Check sheet for the modelled part. Datum: model origin and axes. Units: mm. A direction names the side the tool comes from. Round coordinates to 2 decimals unless told otherwise and drop trailing zeros. Write each loop counter-clockwise with the first axis right and the second up, starting at its lowest first coordinate (ties: lowest second). Pieces come first, ordered by that corner, then holes.
Item 1: Release check for a two-part mould opening along X. For faces 1 (the cylindrical face through (-2.532, -59.947, 12.325)), 2 (the flat face through (0, 51.337, 12)), 3 (the flat face through (39, -13, 25)) record: pulls with the +X half, pulls with the -X half, needs draft (parallel to the pull), parting line crosses it, or undercut.
Item 2: Material ranges on line 1 along Y through (x, z) = (0, 10); line 2 along Y through (x, z) = (-31.5, 21.75); line 3 along X through (y, z) = (-3, 8), recorded low to high.
Item 3: Depth check by flat-ended pin: pin 1 (1.5 mm diameter, centred on y = 45.5, z = 22.5, fed in from -X); pin 2 (3 mm diameter, centred on x = 31, y = 26, fed in from -Z); pin 3 (1.5 mm diameter, centred on y = -29, z = 19.5, fed in from +X); pin 4 (10 mm diameter, centred on y = 35.5, z = 15, fed in from -X). Enter the tip coordinate at first touch or a pass-through.
Item 4: Section check B-B, the plane x = 0. Record the cut outline in (y, z).
Item 5: Section check D-D, the plane y = -49.5. Record the cut outline in (x, z), plus the area to 3 significant figures.
Item 6: Section check A-A, the plane y = 0. Record the cut outline in (x, z).
Item 7: Section check C-C, the plane z = 2. Record the cut outline in (x, y), plus the area to 3 significant figures.
Item 8: Set-up check for faces 4 (the cylindrical face through (-8.67, -39.05, 12.32)), 5 (the flat face through (-5.97, 56.05, 12.32)): record each of +Z, -Z, +X, -X, +Y, -Y from which the full face is reachable in a straight line by a thin tool's end or side.
from build123d import *

# Parameters (mm, degrees)
F0_R     = 60
F0_R_2   = 40
F1_DEPTH = 25
F4_DEPTH = 25.001


with BuildPart() as f1:
    # F0 (on Top) → F1 (new body)
    with BuildSketch(Plane.XY):
        Circle(F0_R)
        Circle(F0_R_2, mode=Mode.SUBTRACT)
    extrude(amount=F1_DEPTH)

    # F3 (on Top) + F2 (on face) → F4 (cut, through all)
    with BuildSketch(Plane.XY):
        with BuildLine():
            ThreePointArc((7.58927, 59.51809), (0, 60.215254), (-7.58927, 59.51809))
            Line((-7.58927, 59.51809), (-4.312616, 52.491282))
            ThreePointArc((-4.312616, 52.491282), (-3.574599, 51.649735), (-2.5, 51.336518))
            Line((-2.5, 51.336518), (2.5, 51.336518))
            ThreePointArc((2.5, 51.336518), (3.574599, 51.649735), (4.312616, 52.491282))
            Line((4.312616, 52.491282), (7.58927, 59.51809))
        make_face()
    with BuildSketch(Plane(origin=(0, 0, 0), x_dir=(1, 0, 0), z_dir=(0, 0, -1))):
        with BuildLine():
            Line((-3.065543, -69.518532), (0, -60))
            ThreePointArc((0, -60), (-11.359106, -58.914945), (-22.307369, -55.699024))
            Line((-22.307369, -55.699024), (-22.307369, -65.699024))
            ThreePointArc((-22.307369, -65.699024), (-14.254384, -75.507649), (-3.065543, -69.518532))
        make_face()
    extrude(amount=F4_DEPTH, mode=Mode.SUBTRACT)


solid = f1.part
Values found:
1. face 1: parting line crosses it
1. face 2: undercut
1. face 3: needs draft
2. line 1: y = -60 to -40, 40 to 51.34
2. line 2: y = -51.07 to -24.65, 24.65 to 51.07
2. line 3: x = -59.92 to -39.89, 39.89 to 59.92
3. pin 1: stops at x = -39.97
3. pin 2: stops at z = 0
3. pin 3: stops at x = 52.93
3. pin 4: stops at x = -51.67
4. outline: (-60, 0) - (-40, 0) - (-40, 25) - (-60, 25) - close; (40, 0) - (51.34, 0) - (51.34, 25) - (40, 25) - close
5. outline: (-33.91, 0) - (33.91, 0) - (33.91, 25) - (-33.91, 25) - close
5. area: 1,700 mm2
6. outline: (-60, 0) - (-40, 0) - (-40, 25) - (-60, 25) - close; (40, 0) - (60, 0) - (60, 25) - (40, 25) - close
7. outline: (-7.59, 59.52) arc R60 ccw (long way) to (7.59, 59.52) - (4.31, 52.49) arc R2 cw to (2.5, 51.34) - (-2.5, 51.34) arc R2 cw to (-4.31, 52.49) - close; hole circle Ø80 at (0, 0)
7. area: 6,190 mm2
8. face 4: +Z, -Z
8. face 5: +Z, -Z, +Y
